Read the model definition and answer for the solid it produces. Units are mm, in the model's axes. A direction names the side the tool comes from. Coordinates: 2 decimals unless noted, no trailing zeros. Loops run counter-clockwise (first coordinate to the right, second up) from the corner with the lowest first, then second, coordinate; pieces in that order, holes last. Notation, with made-up numbers: (34.25, 23) - (74.25, 23) arc R34 ccw to (74.25, 62) - close; hole circle Ø5 at (83.5, 87.25). An arc over 180 degrees is marked (long way). Use one line per item in the form item = value.
from build123d import *

# Parameters (mm, degrees)
SALIENTE_EXTRUIR1_DEPTH  = 21.5
CORTAR_EXTRUIR1_DEPTH    = 8.5
CORTAR_EXTRUIR2_DEPTH    = 3.5000001
CROQUIS5_W               = 12
CROQUIS5_H               = 10.5
SALIENTE_EXTRUIR2_DEPTH  = 4
CROQUIS6_W               = 11
CROQUIS6_H               = 9.5
CORTAR_EXTRUIR3_DEPTH    = 5
CROQUIS8_R               = 2.95
SALIENTE_EXTRUIR8_DEPTH  = 5
CROQUIS9_R               = 0.95
CORTAR_EXTRUIR4_DEPTH    = 5.5
CROQUIS12_R              = 2.9
SALIENTE_EXTRUIR14_DEPTH = 5
CROQUIS13_R              = 0.9
CORTAR_EXTRUIR5_DEPTH    = 5.5


with BuildPart() as part:
    # Croquis1 → Saliente-Extruir1 (new body)
    with BuildSketch(Plane.XY):
        Polygon((-7.838981289, 5.169230769), (13.161018711, 5.169230769), (13.161018711, 3.669230769), (8.961018711, 3.669230769), (8.961018711, 2.669230769), (-26.238981289, 2.669230769), (-26.238981289, 3.669230769), align=None)
    extrude(amount=SALIENTE_EXTRUIR1_DEPTH)

    # Croquis2 → Cortar-Extruir1 (cut)
    with BuildSketch(Plane(origin=(0, 0, 0), x_dir=(-1, 0, 0), z_dir=(0, 0, -1))):
        with BuildLine():
            Line((2.838981289, 5.169230769), (7.838981289, 5.169230769))
            add(Edge.make_bspline(
                [(5.338981289, 4.169230769), (7.838981289, 4.169230769), (7.838981289, 5.169230769)],
                knots=[4.71238898, 4.71238898, 4.71238898, 6.283185307, 6.283185307, 6.283185307], degree=2, weights=[1, 0.707106781, 1]))
            add(Edge.make_bspline(
                [(2.838981289, 5.169230769), (2.838981289, 4.169230769), (5.338981289, 4.169230769)],
                knots=[0, 0, 0, 1.570796327, 1.570796327, 1.570796327], degree=2, weights=[1, 0.707106781, 1]))
        make_face()
    extrude(amount=-CORTAR_EXTRUIR1_DEPTH, mode=Mode.SUBTRACT)

    # Croquis3 → Cortar-Extruir2 (cut, through all)
    with BuildSketch(Plane(origin=(0, 5.169230769, 0), x_dir=(1, 0, 0), z_dir=(0, 1, 0))):
        Polygon((-5.338981289, -8.5), (-10.338981289, -8.5), (-10.338981289, -17), (-0.338981289, -17), (-0.338981289, -8.5), align=None)
    extrude(amount=-CORTAR_EXTRUIR2_DEPTH, mode=Mode.SUBTRACT)

    # Croquis5 → Saliente-Extruir2 (add)
    with BuildSketch(Plane.XZ.offset(-2.669230769)):
        with Locations((-5.338981289, 12.75)):
            Rectangle(CROQUIS5_W, CROQUIS5_H)
    extrude(amount=SALIENTE_EXTRUIR2_DEPTH)

    # Croquis6 → Cortar-Extruir3 (cut)
    with BuildSketch(Plane.XZ.offset(1.330769231)):
        with Locations((-5.338981289, 12.75)):
            Rectangle(CROQUIS6_W, CROQUIS6_H)
    extrude(amount=-CORTAR_EXTRUIR3_DEPTH, mode=Mode.SUBTRACT)

    # Croquis8 → Saliente-Extruir8 (add)
    with BuildSketch(Plane.XZ.offset(-2.669230769)):
        with Locations((3.561018711, 12.75)):
            Circle(CROQUIS8_R)
    extrude(amount=SALIENTE_EXTRUIR8_DEPTH)

    # Croquis9 → Cortar-Extruir4 (cut)
    with BuildSketch(Plane.XZ.offset(2.330769231)):
        with Locations((3.561018711, 12.75)):
            Circle(CROQUIS9_R)
    extrude(amount=-CORTAR_EXTRUIR4_DEPTH, mode=Mode.SUBTRACT)

    # Croquis12 → Saliente-Extruir14 (add)
    with BuildSketch(Plane.XZ.offset(-2.669230769)):
        with Locations((-14.248981289, 12.75)):
            Circle(CROQUIS12_R)
    extrude(amount=SALIENTE_EXTRUIR14_DEPTH)

    # Croquis13 → Cortar-Extruir5 (cut)
    with BuildSketch(Plane.XZ.offset(2.330769231)):
        with Locations((-14.248981289, 12.75)):
            Circle(CROQUIS13_R)
    extrude(amount=-CORTAR_EXTRUIR5_DEPTH, mode=Mode.SUBTRACT)


solid = part.part
Item 1: The part is cut by section D-D on x = -23. Give the vertices of the cut face in (y, z), plus the area to 3 significant figures.
Results below:
outline = (2.67, 0) - (3.93, 0) - (3.93, 21.5) - (2.67, 21.5) - close
area = 27.2 mm²
Item 2: Which of the six approach directions +Z, -Z, +X, -X, +Y, -Y give full straight-line access (tool end or side, diameter ignored) to faces 1 (the flat face through (-6, 4, 21.5)), 2 (the flat face through (0.161, 1, 13)), 3 (the flat face through (11, 3.669, 11)), 4 (the flat face through (-5, 4, 17))?
Results below:
face_1 = +Z, +X, -X, +Y, -Y
face_2 = -Y
face_3 = +Z, -Z, +X, -Y
face_4 = +Y, -Y
Item 3: The part is cut by section A-A on y = -0.5. Give the vertices of the cut face in (x, z), plus the area to 3 significant figures.
Results below:
outline = circle Ø5.8 at (-14.25, 12.75); (-11.34, 7.5) - (0.66, 7.5) - (0.66, 12.21) arc R2.95 ccw (long way) to (0.66, 13.29) - (0.66, 18) - (-11.34, 18) - close; hole circle Ø1.8 at (-14.25, 12.75); hole (-10.84, 8) - (0.16, 8) - (0.16, 17.5) - (-10.84, 17.5) - close; hole circle Ø1.9 at (3.56, 12.75)
area = 69.8 mm²
Item 4: For a pull along X with two mould halves and no side action, classify faces 5 (the flat face through (-6, 4, 0)), 6 (the flat face through (-5, 1, 17.5)), 7 (the flat face through (-14, 3.169, 13)) as +X half, -X half, draft (parallel to the pull), parting line (faces both ways), or undercut.
Results below:
face_5 = draft
face_6 = undercut
face_7 = undercut
Item 5: Each of these flat-tipped pins is pushed along its axis until it touches: P1, Ø2, axis at x = -21.5, z = 15, coming from the -Y side; P2, Ø4, axis at x = -6, y = 1.5, coming from the -Z side; P3, Ø6, axis at x = -14.5, z = 6, coming from the +Y side; P4, Ø4.5, axis at x = -6, y = 0, coming from the -Z side. Where does it stop, or does it pass through?
Results below:
P1 = 2.67
P2 = 0
P3 = 4.87
P4 = 7.5
Item 6: The part is cut by section C-C on x = -18.5. Give the vertices of the cut face in (y, z), plus the area to 3 significant figures.
Results below:
outline = (2.67, 0) - (4.3, 0) - (4.3, 21.5) - (2.67, 21.5) - close
area = 35.1 mm²
Item 7: Find the intervals of material crossed by L1, parallel to X at y = 0.75, z = 15; L2, parallel to X at y = 1.75, z = 10.75; L3, parallel to Z at x = -6, y = 3.25, in increasing order.
Results below:
L1 = -16.08 to -12.42, -11.34 to -10.84, 0.16 to 0.66, 1.65 to 5.47
L2 = -16.35 to -12.15, -11.34 to -10.84, 0.16 to 0.66, 1.39 to 5.73
L3 = 0 to 8, 17.5 to 21.5
